The drawing under review shows one solid part. Ordinate dimensions are in mm from its lowest x, y, z. A direction names the side the tool comes from. Coordinates: 2 decimals unless noted, no trailing zeros. Write each loop counter-clockwise with the first axis right and the second up, starting at its lowest first coordinate (ties: lowest second). Pieces come first, ordered by that corner, then holes.
1) To check wall thickness, follow line 1 along Y through (x, z) = (20, 3.5); line 2 along X through (y, z) = (33, 1.5); line 3 along X through (y, z) = (25.5, 2.25). State the ranges of each line that lie inside material, in increasing order.
2) We need section B-B on y = 10. Write out the cut boundary in (x, z), then the cut area to 3 significant figures.
3) Mouldability with a two-part tool opening along Y and no side actions: class the marked faces 1, 2, 3 and 4 as pulls with the +Y half, pulls with the -Y half, needs draft (parallel to the pull), parting line crosses it, or undercut.
4) We need section A-A on z = 8. Write out the cut boundary in (x, y), then the cut area to 3 significant figures.
5) Insertion check: P1, Ø0.9, axis at x = 33.5, z = 7.5, coming from the -Y side; P2, Ø1.5, axis at x = 35, z = 8, coming from the +Y side; P3, Ø3, axis at y = 43, z = 4.5, coming from the +X side; P4, Ø5, axis at x = 20, y = 10, coming from the +Z side. Each pin has a flat end and moves straight along its axis. Give the tip position at first contact, or say it passes through.
6) We need section D-D on z = 2.75. Write out the cut boundary in (x, y).
7) For the marked faces 5, 6 and 7, list the 3-axis set-ups (+Z, -Z, +X, -X, +Y, -Y) from which the entire face can be reached by the end or side of a thin tool; tool diameter is ignored.
8) We need section C-C on x = 20. Write out the cut boundary in (y, z), then the cut area to 3 significant figures.
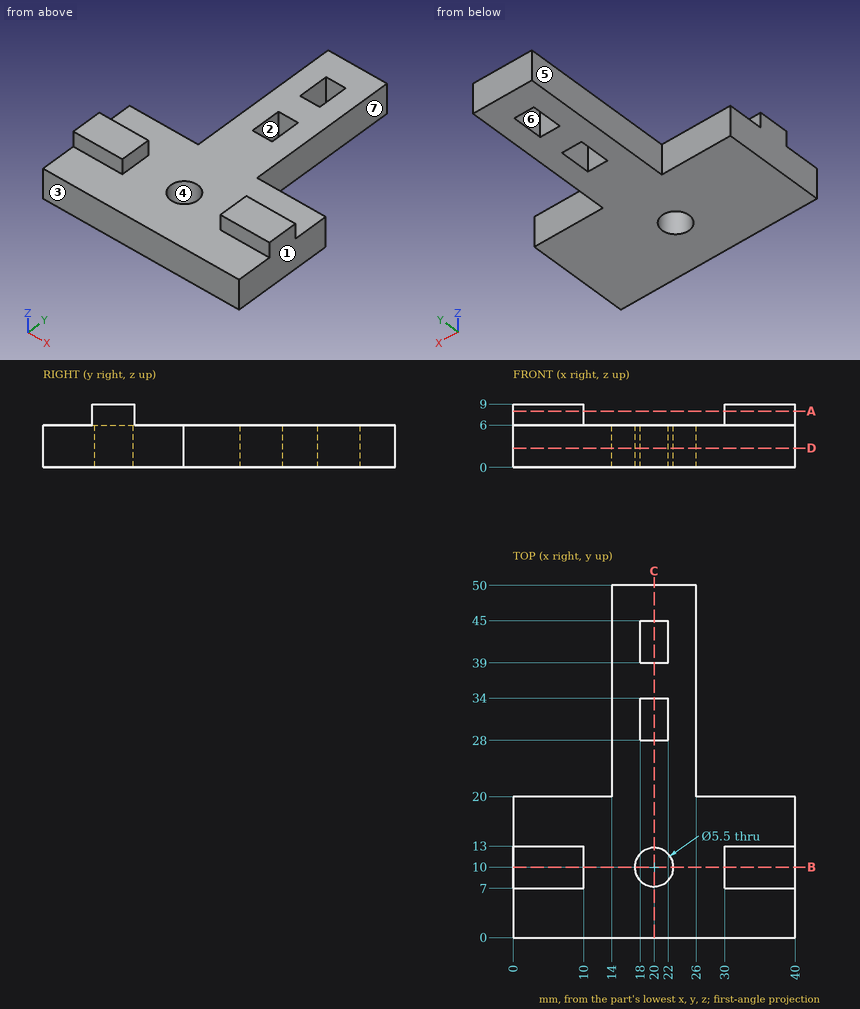
Result:
1. line 1: y = 0 to 7.25, 12.75 to 28, 34 to 39, 45 to 50
1. line 2: x = 14 to 18, 22 to 26
1. line 3: x = 14 to 26
2. outline: (0, 0) - (17.25, 0) - (17.25, 6) - (10, 6) - (10, 9) - (0, 9) - close; (22.75, 0) - (40, 0) - (40, 9) - (30, 9) - (30, 6) - (22.75, 6) - close
2. area: 267 mm2
3. face 1: needs draft
3. face 2: undercut
3. face 3: pulls with the -Y half
3. face 4: undercut
4. outline: (0, 7) - (10, 7) - (10, 13) - (0, 13) - close; (30, 7) - (40, 7) - (40, 13) - (30, 13) - close
4. area: 120 mm2
5. P1: stops at y = 7
5. P2: stops at y = 13
5. P3: stops at x = 26
5. P4: passes through
6. outline: (0, 0) - (40, 0) - (40, 20) - (26, 20) - (26, 50) - (14, 50) - (14, 20) - (0, 20) - close; hole circle Ø5.5 at (20, 10); hole (18, 28) - (22, 28) - (22, 34) - (18, 34) - close; hole (18, 39) - (22, 39) - (22, 45) - (18, 45) - close
7. face 5: +Z, -Z, -X, +Y
7. face 6: +Z, -Z
7. face 7: +Z, -Z, +X, +Y
8. outline: (0, 0) - (7.25, 0) - (7.25, 6) - (0, 6) - close; (12.75, 0) - (28, 0) - (28, 6) - (12.75, 6) - close; (34, 0) - (39, 0) - (39, 6) - (34, 6) - close; (45, 0) - (50, 0) - (50, 6) - (45, 6) - close
8. area: 195 mm2
